Job drawing, mm, ordinate dimensions from the low corner. One solid piece. A direction names the side the tool comes from. Round coordinates to 2 decimals unless told otherwise and drop trailing zeros. Write each loop counter-clockwise with the first axis right and the second up, starting at its lowest first coordinate (ties: lowest second). Pieces come first, ordered by that corner, then holes.
1) Saw through at A-A (y = 21). Write the cut outline in (x, z).
2) Flat gauge pins, fed straight in: pin 1 (10 mm diameter, centred on y = 34.5, z = 48.5, fed in from -X); pin 2 (8 mm diameter, centred on x = 30, y = 37.5, fed in from +Z). Where does each tip first touch, or does it go through?
3) Wall check: probe 1 along Z at (x, y) = (35.5, 40); probe 2 along X at (y, z) = (2.5, 12.5); probe 3 along Y at (x, z) = (17.5, 47). Give the ranges that are in metal, low to high.
4) Saw through at B-B (x = 22). Write the cut outline in (y, z), plus the area to 3 significant figures.
5) Saw through at D-D (x = 7.5). Write the cut outline in (y, z), plus the area to 3 significant figures.
6) Which spindle directions (+Z, -Z, +X, -X, +Y, -Y) get a long thin tool onto all of the face, cutting with end or side? Do the marked faces 1 and 2. Say none if no direction does.
7) Saw through at C-C (z = 41). Write the cut outline in (x, y), plus the area to 3 significant figures.
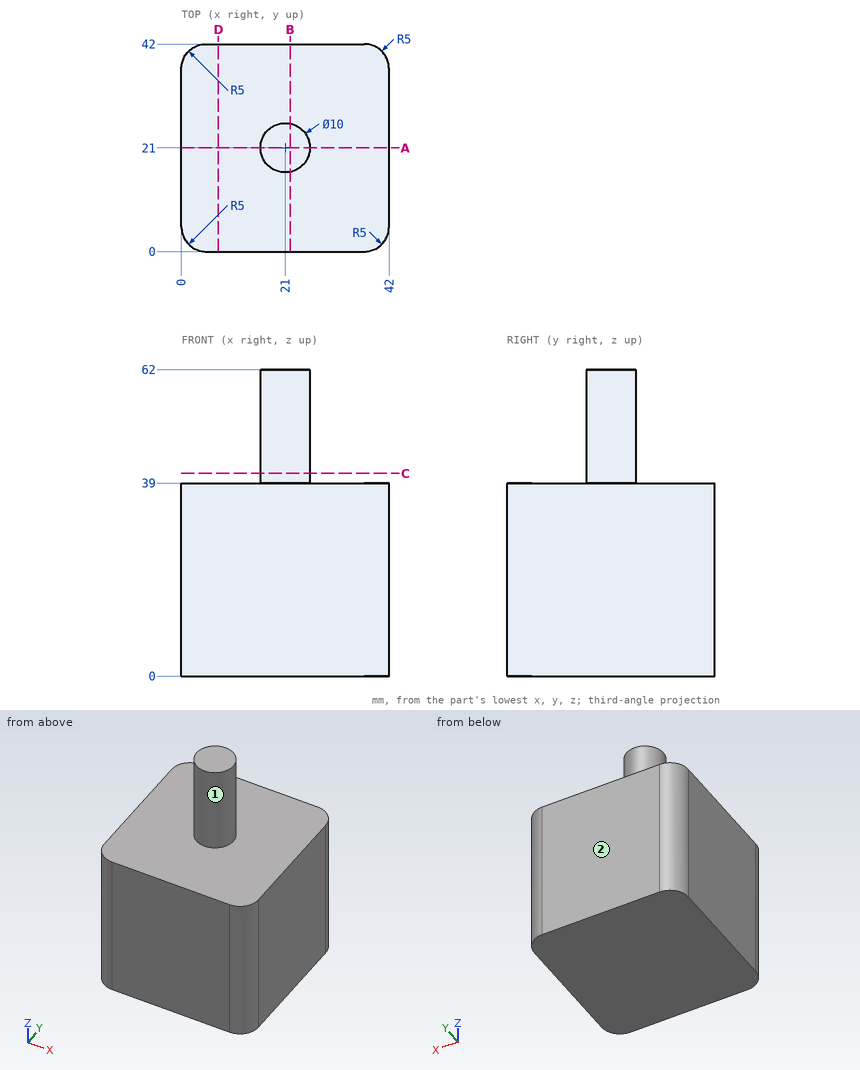
Evaluation:
1. outline: (0, 0) - (42, 0) - (42, 39) - (26, 39) - (26, 62) - (16, 62) - (16, 39) - (0, 39) - close
2. pin 1: passes through
2. pin 2: stops at z = 39
3. probe 1: z = 0 to 39
3. probe 2: x = 0.67 to 41.33
3. probe 3: y = 17.43 to 24.57
4. outline: (0, 0) - (42, 0) - (42, 39) - (25.9, 39) - (25.9, 62) - (16.1, 62) - (16.1, 39) - (0, 39) - close
4. area: 1,860 mm2
5. outline: (0, 0) - (42, 0) - (42, 39) - (0, 39) - close
5. area: 1,640 mm2
6. face 1: +Z
6. face 2: +Z, -Z, +X, -X, +Y
7. outline: circle Ø10 at (21, 21)
7. area: 78.5 mm2
